from build123d import *

# Parameters (mm, degrees)
F0_R     = 63.5
F1_DEPTH = 19.05
F2_R     = 6.35
F3_DEPTH = 381
F4_R     = 6.35
F5_DEPTH = 381


with BuildPart() as f1:
    # F0 (on Top) → F1 (new body, symmetric)
    with BuildSketch(Plane.XY):
        Circle(F0_R)
    extrude(amount=F1_DEPTH, both=True)

    # F2 (on Front) → F3 (cut, symmetric)
    with BuildSketch(Plane.XZ):
        Circle(F2_R)
    extrude(amount=F3_DEPTH, both=True, mode=Mode.SUBTRACT)

    # F4 (on Right) → F5 (cut, symmetric)
    with BuildSketch(Plane.YZ):
        Circle(F4_R)
    extrude(amount=F5_DEPTH, both=True, mode=Mode.SUBTRACT)


solid = f1.part
The model under review builds one solid part; all positions refer to its coordinate system, in mm. Give positions to 0.01 mm unless a question says otherwise; leave off trailing zeros. Order: outer loops, then holes, each group sorted by start corner. A loop starts at its lowest first (then second) coordinate and runs counter-clockwise, first axis right, second up. Notation, with made-up numbers: M 57,-36 L 108,-36 A8 ccw 108,-21 Z; hole C 1,6 d11. An arc over 180 degrees is marked long. Use one line per item in the form item = value. Start each with the question number.
Item 1: We need section D-D on y = 43. Give the boundary of the cut face in (x, z).
Item 2: Insertion check: pin 1 Ø5 at (x, z) = (-1.5, -11.5) entering from -Y; pin 2 Ø1 at (y, z) = (17.5, 14.5) entering from -X; pin 3 Ø5 at (y, z) = (-47.5, -5.5) entering from +X; pin 4 Ø5 at (y, z) = (6, 0) entering from -X. Each pin has a flat end and moves straight along its axis. Give the tip position at first contact, or say it passes through.
Item 3: We need section C-C on y = -3.5. Give the boundary of the cut face in (x, z), plus the area to 3 significant figures.
Item 4: We need section B-B on z = -4. Give the boundary of the cut face in (x, y), plus the area to 3 significant figures.
Item 5: The part is to be moulded in two halves that separate along Y. For faces 1 (the cylindrical face through (32.194, 6.057, 1.907)), 2 (the cylindrical face through (58.66, -24.32, 0.27)), 3 (the flat face through (-1, 1, -19.05)), say which applies: pulls with the +Y half, pulls with the -Y half, needs draft (parallel to the pull), parting line crosses it, or undercut.
Item 6: We need section A-A on x = 4.5. Give the boundary of the cut face in (y, z).
Item 7: To check wall thickness, follow line 1 along Z through (x, y) = (43, 0); line 2 along Y through (x, z) = (15.5, 0); line 3 along Y through (x, z) = (30, 0). State the ranges of each line that lie inside material, in increasing order. Write a range as from..to.
Completed:
q1.outline = M -46.73,-19.05 L 46.73,-19.05 L 46.73,19.05 L -46.73,19.05 Z; hole C 0,0 d12.7
q2.pin_1 = -63.5
q2.pin_2 = -61.18
q2.pin_3 = 44.8
q2.pin_4 = -63.23
q3.outline = M -63.4,-19.05 L 63.4,-19.05 L 63.4,-5.3 L 3.5,-5.3 A6.35 cw -3.5,-5.3 L -63.4,-5.3 Z; M -63.4,5.3 L -3.5,5.3 A6.35 cw 3.5,5.3 L 63.4,5.3 L 63.4,19.05 L -63.4,19.05 Z
q3.area = 3,480 mm²
q4.outline = M -63.31,-4.93 A63.5 ccw -4.93,-63.31 L -4.93,-4.93 Z; M -63.31,4.93 L -4.93,4.93 L -4.93,63.31 A63.5 ccw Z; M 4.93,-63.31 A63.5 ccw 63.31,-4.93 L 4.93,-4.93 Z; M 4.93,4.93 L 63.31,4.93 A63.5 ccw 4.93,63.31 Z
q4.area = 10,300 mm²
q5.face_1 = undercut
q5.face_2 = parting line crosses it
q5.face_3 = needs draft
q6.outline = M -63.34,-19.05 L 63.34,-19.05 L 63.34,-4.48 L 4.5,-4.48 A6.35 cw -4.5,-4.48 L -63.34,-4.48 Z; M -63.34,4.48 L -4.5,4.48 A6.35 cw 4.5,4.48 L 63.34,4.48 L 63.34,19.05 L -63.34,19.05 Z
q7.line_1 = -19.05..-6.35, 6.35..19.05
q7.line_2 = -61.58..-6.35, 6.35..61.58
q7.line_3 = -55.97..-6.35, 6.35..55.97
